The model under review builds one solid part; all positions refer to its coordinate system, in mm. Give positions to 0.01 mm unless a question says otherwise; leave off trailing zeros. Write each loop counter-clockwise with the first axis right and the second up, starting at its lowest first coordinate (ties: lowest second). Pieces come first, ordered by that corner, then holes. Notation, with made-up numbers: (-9, 28.5) - (0, 28.5) arc R13 ccw to (0, 51.5) - close; hole circle Ø3 at (58, -21). An arc over 180 degrees is marked (long way). One line per question, with ' | ' between items. Start each with the question number.
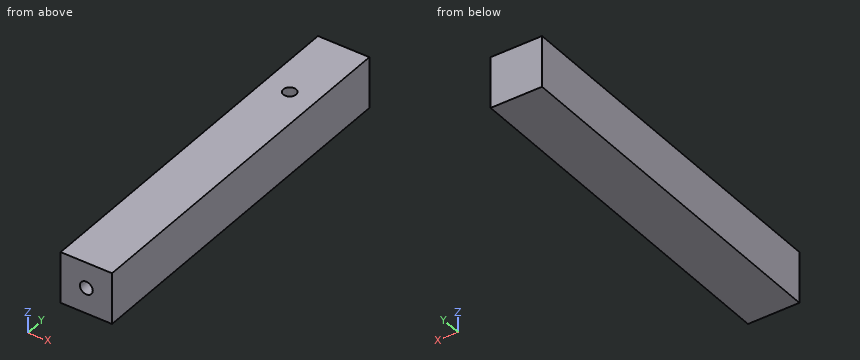
Autodesk Inventor part; units mm, degrees
ref_plane "YZ Plane" through (0, 0, 0) normal (1, 0, 0) x (0, 1, 0)
ref_plane "XZ Plane" through (0, 0, 0) normal (0, 1, 0) x (-1, 0, 0)
ref_plane "XY Plane" through (0, 0, 0) normal (0, 0, 1) x (1, 0, 0)
sketch "Boceto1" plane through (0, 0, 0) normal (0, 0, 1) x (1, 0, 0)
  line L0 (-10, -71.5) -> (10, -71.5)
  line L1 (10, -71.5) -> (10, 71.5)
  line L2 (10, 71.5) -> (-10, 71.5)
  line L3 (-10, 71.5) -> (-10, -71.5)
  line L4 (-10, -71.5) -> (10, 71.5) construction
  line L5 (10, -71.5) -> (-10, 71.5) construction
  point P0 (0, 0)
  dimension "d0" = 20
  dimension "d1" = 143
extrude "Extrusión1" add sketch "Boceto1" against normal blind 20
sketch "Boceto2" plane through (0, 0, 0) normal (0, 0, 1) x (1, 0, 0)
  line L0 (-10, 71.5) -> (10, 71.5)
  circle A0 centre (0, 41.5) radius 2.5
  point P0 (0, 0)
  dimension "d5" = 5
extrude "Extrusión2" cut sketch "Boceto2" against normal blind 10
thread "Rosca1"
sketch "Boceto3" plane through (-10, -71.5, 0) normal (0, -1, 0) x (1, 0, 0)
  circle A0 centre (10, -10) radius 2.5
  point P0 (10, 0)
extrude "Extrusión3" cut sketch "Boceto3" against normal blind 10
thread "Rosca2"
properties part number "Suport_Cam"
Item 1: Take a section at A-A (x = 0). Give the boundary of the cut face in (y, z), plus the area to 3 significant figures.
Item 2: Clearance check with a flat-ended pin moving along its axis: P1, Ø4.5, axis at x = 0, y = 41.5, coming from the +Z side. State where the tip first meets the part, or that it passes through.
Item 3: For probe 1 along Z at (x, y) = (0, -67.75); probe 2 along Y at (x, z) = (0, -4.75); probe 3 along Y at (x, z) = (-1.5, -8.5), list the stretches that pass through material, from the lowest coordinate up.
Item 4: Take a section at B-B (y = 41.5). Give the boundary of the cut face in (x, z), plus the area to 3 significant figures.
Check sheet entries:
1) outline: (-71.5, -20) - (71.5, -20) - (71.5, 0) - (44, 0) - (44, -10) - (39, -10) - (39, 0) - (-71.5, 0) - (-71.5, -7.5) - (-61.5, -7.5) - (-61.5, -12.5) - (-71.5, -12.5) - close | area: 2,760 mm^2
2) P1: stops at z = -10
3) probe 1: z = -20 to -12.5, -7.5 to 0 | probe 2: y = -71.5 to 39, 44 to 71.5 | probe 3: y = -61.5 to 39.5, 43.5 to 71.5
4) outline: (-10, -20) - (10, -20) - (10, 0) - (2.5, 0) - (2.5, -10) - (-2.5, -10) - (-2.5, 0) - (-10, 0) - close | area: 350 mm^2
